```python
from build123d import *

# Parameters (mm, degrees)
SKETCH2_R              = 14.2875
BOSS_EXTRUDE1_DEPTH    = 3.175
SKETCH3_W              = 44.45
SKETCH3_H              = 3.175
BOSS_EXTRUDE2_DEPTH    = 25.4
SKETCH4_R              = 2.032
CUT_EXTRUDE1_DEPTH     = 25.4
FILLET1_R              = 2.54
CONVERT_SOLID1_START   = -22.225
CONVERT_SOLID1_DEPTH   = 44.45
CONVERT_SOLID1_2_DEPTH = 44.45


# Read off the part's stored shape, not the designer's step: Convert-Solid1
with BuildPart() as part:
    # Sketch2 → Boss-Extrude1 (new body)
    with BuildSketch(Plane.XY):
        with BuildLine():
            Line((-22.225, -19.05), (22.225, -19.05))
            Line((22.225, -19.05), (22.225, 16.51))
            ThreePointArc((22.225, 16.51), (21.481051224, 18.306051224), (19.685, 19.05))
            Line((19.685, 19.05), (-19.685, 19.05))
            ThreePointArc((-19.685, 19.05), (-21.481051224, 18.306051224), (-22.225, 16.51))
            Line((-22.225, 16.51), (-22.225, -19.05))
        make_face()
        Circle(SKETCH2_R, mode=Mode.SUBTRACT)
    extrude(amount=BOSS_EXTRUDE1_DEPTH)

    # Sketch3 → Boss-Extrude2 (add)
    with BuildSketch(Plane(origin=(0, 0, 0), x_dir=(-1, 0, 0), z_dir=(0, 0, -1))):
        with Locations((0, -17.4625)):
            Rectangle(SKETCH3_W, SKETCH3_H)
    extrude(amount=BOSS_EXTRUDE2_DEPTH)

    # Sketch4 → Cut-Extrude1 (cut)
    with BuildSketch(Plane(origin=(0, -15.875, 0), x_dir=(1, 0, 0), z_dir=(0, 1, 0))):
        with Locations(Location((-9.525, 12.7, 0), (0, 0, 270))):
            Circle(SKETCH4_R)
        with Locations(Location((9.525, 12.7, 0), (0, 0, 270))):
            Circle(SKETCH4_R)
    extrude(amount=-CUT_EXTRUDE1_DEPTH, mode=Mode.SUBTRACT)

    # Fillet1
    fillet1_edges = [part.edges().sort_by_distance(p)[0] for p in [
        (22.225, -17.4625, -25.4),
        (-22.225, -17.4625, -25.4),
    ]]
    fillet(fillet1_edges, radius=FILLET1_R)

    # Convert-Solid1 outline → Convert-Solid1 (cut)
    with BuildSketch(Plane.YZ.offset(CONVERT_SOLID1_START)):
        with BuildLine():
            ThreePointArc((-19.05, -1.27), (-17.748089642, 1.873089642), (-14.605, 3.175))
            Line((-14.605, 3.175), (-19.05, 3.175))
            Line((-19.05, 3.175), (-19.05, -1.27))
        make_face()
    extrude(amount=CONVERT_SOLID1_DEPTH, mode=Mode.SUBTRACT)

    # Convert-Solid1 2 outline → Convert-Solid1 2 (add)
    with BuildSketch(Plane.YZ.offset(CONVERT_SOLID1_START)):
        with BuildLine():
            ThreePointArc((-15.875, -1.27), (-15.503025612, -0.371974388), (-14.605, 0))
            Line((-14.605, 0), (-15.875, 0))
            Line((-15.875, 0), (-15.875, -1.27))
        make_face()
    extrude(amount=CONVERT_SOLID1_2_DEPTH)


solid = part.part
```
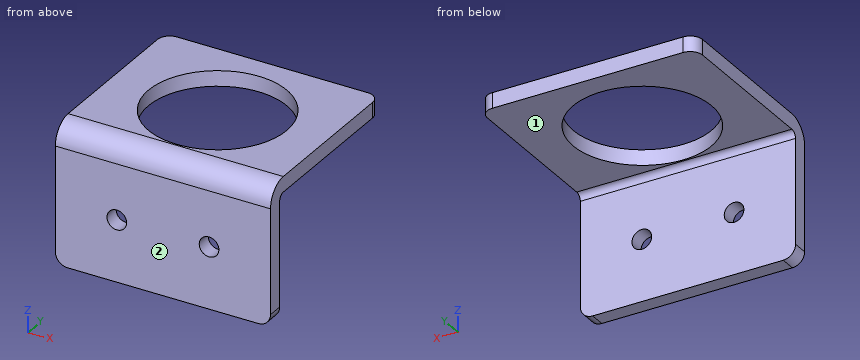
Here's how the part is built. I have some questions about the finished solid (model axes, mm). Face numbers are marked on the shaded views. A direction names the side the tool comes from. Coordinates: 2 decimals unless noted, no trailing zeros. Loops run counter-clockwise (first coordinate to the right, second up) from the corner with the lowest first, then second, coordinate; pieces in that order, holes last. Notation, with made-up numbers: (63.5, -10.5) -> (94.5, -10.5) arc R24 ccw to (94.5, 23.5) -> close; hole circle Ø9 at (32.5, -22). An arc over 180 degrees is marked (long way). Return JSON: item names as keys, results as strings.
1) Will these pins go through, and if not, where does the flat tip stop? pin 1 (2 mm diameter, centred on x = 2.5, z = -4.5, fed in from +Y) (3 decimals); pin 2 (3.5 mm diameter, centred on x = 9.525, z = -12.7, fed in from -Y); pin 3 (5 mm diameter, centred on y = 6.5, z = -2, fed in from -X) (3 decimals); pin 4 (12 mm diameter, centred on x = -11, y = 6, fed in from -Z).
Results below:
{"pin 1": "y = -15.875", "pin 2": "through", "pin 3": "x = -22.225", "pin 4": "z = 0"}
2) If we section it at C-C, the plane z = -12.7: Write out the boundary of the cut face in (x, y) (3 decimals).
Results below:
{"outline": "(-22.225, -19.05) -> (-11.557, -19.05) -> (-11.557, -15.875) -> (-22.225, -15.875) -> close; (-7.493, -19.05) -> (7.493, -19.05) -> (7.493, -15.875) -> (-7.493, -15.875) -> close; (11.557, -19.05) -> (22.225, -19.05) -> (22.225, -15.875) -> (11.557, -15.875) -> close"}
3) For the marked faces 1 and 2, which set-ups out of +Z, -Z, +X, -X, +Y, -Y let a thin tool reach every point of the face, with its end or its side?
Results below:
{"face 1": "-Z, +X, -X, +Y", "face 2": "+Z, -Z, +X, -X, -Y"}
4) If we section it at A-A, the plane y = 0: Write out the boundary of the cut face in (x, z) (1 decimal).
Results below:
{"outline": "(-22.2, 0) -> (-14.3, 0) -> (-14.3, 3.2) -> (-22.2, 3.2) -> close; (14.3, 0) -> (22.2, 0) -> (22.2, 3.2) -> (14.3, 3.2) -> close"}
5) I need wall thicknesses on line 1 (X direction, y = -17.1, z = -12.7) (3 decimals); line 2 (Y direction, x = -14.5, z = -16.75) (3 decimals); line 3 (Z direction, x = 13.5, y = 16) (3 decimals). Which ranges of each line are inside material? Lowest first, please. Write a range as from..to.
Results below:
{"line 1": "-22.225..-11.557, -7.493..7.493, 11.557..22.225", "line 2": "-19.05..-15.875", "line 3": "0..3.175"}
6) If we section it at D-D, the plane x = -9: Write out the boundary of the cut face in (y, z) (3 decimals).
Results below:
{"outline": "(-19.05, -25.4) -> (-15.875, -25.4) -> (-15.875, -14.663) -> (-19.05, -14.663) -> close; (-19.05, -10.737) -> (-15.875, -10.737) -> (-15.875, -1.27) arc R1.27 cw to (-14.605, 0) -> (-11.097, 0) -> (-11.097, 3.175) -> (-14.605, 3.175) arc R4.445 ccw to (-19.05, -1.27) -> close; (11.097, 0) -> (19.05, 0) -> (19.05, 3.175) -> (11.097, 3.175) -> close"}
